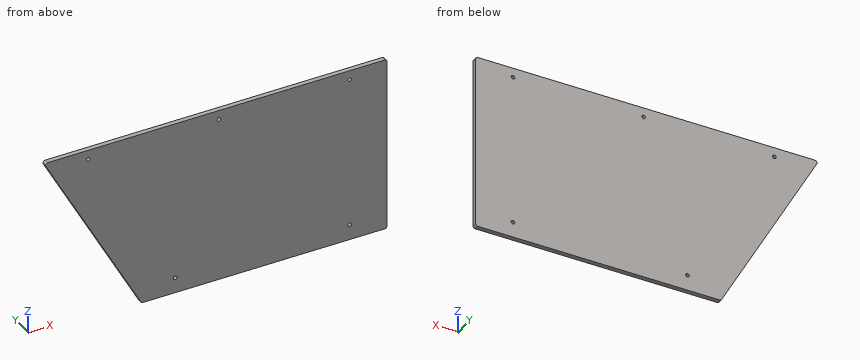
from build123d import *

# Parameters (mm, degrees)
SKETCH1_R           = 2.45745
BOSS_EXTRUDE1_DEPTH = 6.35
FILLET1_R           = 3.175


with BuildPart() as part:
    # Sketch1 → Boss-Extrude1 (new body)
    with BuildSketch(Plane(origin=(0, 0, 0), x_dir=(1, 0, 0), z_dir=(0, 1, 0))):
        Polygon((0, 0), (132.810986877, 238.125), (466.725, 238.125), (466.725, 0), align=None)
        with Locations((415.925, 217.297)):
            Circle(SKETCH1_R, mode=Mode.SUBTRACT)
        with Locations((415.925, 12.7)):
            Circle(SKETCH1_R, mode=Mode.SUBTRACT)
        with Locations((238.125, 12.7)):
            Circle(SKETCH1_R, mode=Mode.SUBTRACT)
        with Locations((60.325, 12.7)):
            Circle(SKETCH1_R, mode=Mode.SUBTRACT)
        with Locations((178.449400022, 217.297)):
            Circle(SKETCH1_R, mode=Mode.SUBTRACT)
    extrude(amount=BOSS_EXTRUDE1_DEPTH)

    # Fillet1
    fillet1_edges = [part.edges().sort_by_distance(p)[0] for p in [
        (0, 3.175, 0),
        (132.810986877, 3.175, -238.125),
        (466.725, 3.175, -238.125),
        (466.725, 3.175, 0),
    ]]
    fillet(fillet1_edges, radius=FILLET1_R)


solid = part.part
Input: part model. Units: mm. Frame: model coordinates. Give positions to 0.01 mm unless a question says otherwise; leave off trailing zeros. Write each loop counter-clockwise with the first axis right and the second up, starting at its lowest first coordinate (ties: lowest second). Pieces come first, ordered by that corner, then holes. Notation, with made-up numbers: M -1,78 L 17,78 A35 ccw 17,115 Z; hole C 76.25,10 d8. An arc over 180 degrees is marked long. Write item = value, one per line. Start each with the question number.
1) Cut plane A-A on y = 4.25. Return the cut outline in (x, z) (3 decimals), then the cut area to 3 significant figures.
2) Cut plane C-C on x = 86. Return the cut outline in (y, z).
3) First-contact query: pin 1 Ø1.5 at (x, y) = (60.5, 1.5) entering from -Z. Flat tip, straight axial feed; report the tip coordinate or a pass-through.
4) Material intervals for line 1 along X through (y, z) = (4.5, -11.5) (3 decimals); line 2 along X through (y, z) = (4.25, -12.7) (3 decimals); line 3 along X through (y, z) = (2, -138) (3 decimals), sorted ascending. Write a range as [from, to].
5) Cut plane B-B on z = -149.5. Return the cut outline in (x, y) (3 decimals).
Solved:
q1.outline = M 2.633,-4.722 L 131.903,-236.497 A3.175 ccw 134.676,-238.125 L 463.55,-238.125 A3.175 ccw 466.725,-234.95 L 466.725,-3.175 A3.175 ccw 463.55,0 L 5.406,0 A3.175 ccw Z; hole C 60.325,-12.7 d4.915; hole C 178.449,-217.297 d4.915; hole C 238.125,-12.7 d4.915; hole C 415.925,-217.297 d4.915; hole C 415.925,-12.7 d4.915
q1.area = 95,200 mm2
q2.outline = M 0,-154.19 L 6.35,-154.19 L 6.35,0 L 0,0 Z
q3.pin_1 = -109.82
q4.line_1 = [6.414, 58.18], [62.47, 235.98], [240.27, 413.78], [418.07, 466.725]
q4.line_2 = [7.083, 57.868], [62.782, 235.668], [240.582, 413.468], [418.382, 466.725]
q4.line_3 = [76.968, 466.725]
q5.outline = M 83.382,0 L 466.725,0 L 466.725,6.35 L 83.382,6.35 Z
